Design review of the part built by this model. Coordinates are the model's own, in mm. A direction names the side the tool comes from. Round coordinates to 2 decimals unless told otherwise and drop trailing zeros. Order: outer loops, then holes, each group sorted by start corner. A loop starts at its lowest first (then second) coordinate and runs counter-clockwise, first axis right, second up. Notation, with made-up numbers: M -11,66 L 36,66 A25 ccw 36,82 Z; hole C 46,68.25 d1. An arc over 180 degrees is marked long. Use a Markdown table: item, result. Add a question column.
(1) Take a section at A-A (y = -10.5). Write out the cut boundary in (x, z).
(2) Take a section at B-B (z = -0.3). Write out the cut boundary in (x, y), then the cut area to 3 significant figures.
(3) Take a section at C-C (x = -1.25). Write out the cut boundary in (y, z), then the cut area to 3 significant figures.
(4) Take a section at D-D (z = 1.65). Write out the cut boundary in (x, y), then the cut area to 3 significant figures.
(5) For pin 1 (1 mm diameter, centred on x = 14, z = 0, fed in from +Y), flat-tipped, find the tip position at first contact; note if it passes through.
(6) Machinability: for faces 1 (the face through (0.137, -0.308, -0.507)), 2 (the face through (10, 0, 0)), 3 (the face through (14.162, -2.466, 0.3)), 4 (the face through (2.338, -2.466, 0.3)), which of the approach directions +Z, -Z, +X, -X, +Y, -Y give a long, thin tool a straight path to every point of the face, cutting with its end or side? Answer none if there is none.
(7) To check wall thickness, follow probe 1 along Z at (x, y) = (1.5, -0.75); probe 2 along X at (y, z) = (-7.5, 1.75); probe 3 along X at (y, z) = (-9, 0.1). State the ranges of each line that lie inside material, in increasing order. Write a range as from..to.
```python
from build123d import *

# Parameters (mm, degrees)
F0_W     = 16.5
F0_H     = 12
F1_DEPTH = 2.5
F2_R     = 8.2
F3_W     = 22.5
F3_H     = 15
F4_DEPTH = 1
F5_R     = 11
F6_SIZE2 = 1.9081136688
F6_SIZE  = 0.1


with BuildPart() as f1:
    # F0 (on Top) → F1 (new body)
    with BuildSketch(Plane.XY):
        with Locations((8.25, -6)):
            Rectangle(F0_W, F0_H)
    extrude(amount=F1_DEPTH)

    # F2
    f2_edges = [f1.edges().sort_by_distance(p)[0] for p in [
        (16.5, 0, 1.25),
        (0, 0, 1.25),
    ]]
    fillet(f2_edges, radius=F2_R)

    # F3 (on face) → F4 (join)
    with BuildSketch(Plane(origin=(0, 0, 0), x_dir=(1, 0, 0), z_dir=(0, 0, -1))):
        with Locations((8.25, 4.5)):
            Rectangle(F3_W, F3_H)
    extrude(amount=F4_DEPTH)

    # F5
    f5_edges = [f1.edges().sort_by_distance(p)[0] for p in [
        (19.5, 3, -0.5),
        (-3, 3, -0.5),
    ]]
    fillet(f5_edges, radius=F5_R)

    # F6
    f6_edges = [f1.edges().sort_by_distance(p)[0] for p in [
        (0, -10.1, 2.5),
        (2.401724, -2.401724, 2.5),
        (14.098276, -2.401724, 2.5),
        (16.5, -10.1, 2.5),
    ]]
    f6_side = f1.faces().sort_by_distance((8.25, -6.711232, 2.5))[0]
    chamfer(f6_edges, length=F6_SIZE, length2=F6_SIZE2, reference=f6_side)


solid = f1.part
```
Verdict:
| question | item | result |
|---|---|---|
| 1 | outline | M -3,-1 L 19.5,-1 L 19.5,0 L 16.5,0 L 16.5,0.59 L 16.4,2.5 L 0.1,2.5 L 0,0.59 L 0,0 L -3,0 Z |
| 2 | outline | M -3,-12 L 19.5,-12 L 19.5,-8 A11 ccw 8.5,3 L 8,3 A11 ccw -3,-8 Z |
| 2 | area | 286 mm^2 |
| 3 | outline | M -12,-1 L -2.05,-1 L -2.05,0 L -12,0 Z |
| 3 | area | 9.95 mm^2 |
| 4 | outline | M 0.06,-12 L 16.44,-12 L 16.44,-8.2 A8.14 ccw 8.3,-0.06 L 8.2,-0.06 A8.14 ccw 0.06,-8.2 Z |
| 4 | area | 167 mm^2 |
| 5 | pin 1 | stops at y = 1.8 |
| 6 | face 1 | +Z, -Z, -X, +Y |
| 6 | face 2 | +Z, +Y |
| 6 | face 3 | +Z, +X, +Y |
| 6 | face 4 | +Z, -X, +Y |
| 7 | probe 1 | z = -1..0 |
| 7 | probe 2 | x = 0.09..16.41 |
| 7 | probe 3 | x = 0..16.5 |
